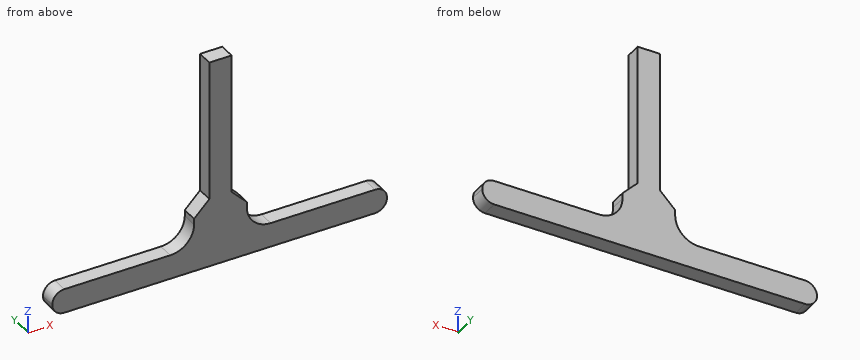
```python
from build123d import *

# Parameters (mm, degrees)
PAD002_DEPTH = 4
FILLET005_R  = 3
FILLET006_R  = 6


with BuildPart() as part:
    # Sketch003 → Pad002 (new body)
    with BuildSketch(Plane.XZ.offset(25)):
        Polygon((-4.149489, 3.072018), (31.436102, 3.072018), (31.436102, 10.54521), (35.263586, 14.418702), (35.263586, 49.841579), (40.852331, 49.841579), (40.852331, 14.418702), (44.676023, 10.554439), (44.676023, 3.072018), (79.850511, 3.072018), (79.850511, -3.027098), (-4.149489, -3.027098), align=None)
    extrude(amount=PAD002_DEPTH)

    # Fillet005
    fillet005_edges = [part.edges().sort_by_distance(p)[0] for p in [
        (79.850511, -27, 3.072018),
        (79.850511, -27, -3.027098),
        (-4.149489, -27, -3.027098),
        (-4.149489, -27, 3.072018),
    ]]
    fillet(fillet005_edges, radius=FILLET005_R)

    # Fillet006
    fillet006_edges = [part.edges().sort_by_distance(p)[0] for p in [
        (44.676023, -27, 3.072018),
        (31.436102, -27, 3.072018),
    ]]
    fillet(fillet006_edges, radius=FILLET006_R)


solid = part.part
```
Build history of the part. All positions in model axes, mm. Coordinates: 2 decimals unless noted, no trailing zeros. Write each loop counter-clockwise with the first axis right and the second up, starting at its lowest first coordinate (ties: lowest second). Pieces come first, ordered by that corner, then holes.
1. Drill centre lines: probe 1 along X at (y, z) = (-27.3, 39); probe 2 along Z at (x, y) = (55, -26.7); probe 3 along X at (y, z) = (-27, 9). Where is each one in solid material? Low to high.
Answer block:
probe 1: x = 35.26 to 40.85
probe 2: z = -3.03 to 3.07
probe 3: x = 31.44 to 44.68
2. Band-saw the part on C-C, the plane x = 57.5. Give the cut face in (y, z), and give its area (3 significant figures).
Answer block:
outline: (-29, -3.03) - (-25, -3.03) - (-25, 3.07) - (-29, 3.07) - close
area: 24.4 mm2
3. Band-saw the part on B-B, the plane z = 25.5. Give the cut face in (x, y).
Answer block:
outline: (35.26, -29) - (40.85, -29) - (40.85, -25) - (35.26, -25) - close
4. Drop flat-ended pins along their axis: pin 1 (1.6 mm diameter, centred on y = -27, z = 10, fed in from -X); pin 2 (1.5 mm diameter, centred on x = 53, y = -27.5, fed in from +Z); pin 3 (1.5 mm diameter, centred on y = -25.5, z = 17.5, fed in from +X). Give the stop position or say it passes through.
Answer block:
pin 1: stops at x = 31.44
pin 2: stops at z = 3.07
pin 3: stops at x = 40.85
5. Band-saw the part on A-A, the plane y = -26.15. Give the cut face in (x, z).
Answer block:
outline: (-4.15, -0.03) arc R3 ccw to (-1.15, -3.03) - (76.85, -3.03) arc R3 ccw to (79.85, -0.03) - (79.85, 0.07) arc R3 ccw to (76.85, 3.07) - (50.68, 3.07) arc R6 cw to (44.68, 9.07) - (44.68, 10.55) - (40.85, 14.42) - (40.85, 49.84) - (35.26, 49.84) - (35.26, 14.42) - (31.44, 10.55) - (31.44, 9.07) arc R6 cw to (25.44, 3.07) - (-1.15, 3.07) arc R3 ccw to (-4.15, 0.07) - close
